Input: part model. Units: mm. Frame: model coordinates. A direction names the side the tool comes from. Give positions to 0.01 mm unless a question says otherwise; leave off trailing zeros. Write each loop counter-clockwise with the first axis right and the second up, starting at its lowest first coordinate (ties: lowest second). Pieces come first, ordered by that corner, then holes.
Autodesk Inventor part; units mm, degrees
ref_plane "YZ Plane" through (0, 0, 0) normal (1, 0, 0) x (0, 1, 0)
ref_plane "XZ Plane" through (0, 0, 0) normal (0, 1, 0) x (-1, 0, 0)
ref_plane "XY Plane" through (0, 0, 0) normal (0, 0, 1) x (1, 0, 0)
sketch "Sketch1" plane through (0, 0, 0) normal (0, 1, 0) x (-1, 0, 0)
  line L0 (25, 0) -> (-25, 0)
  line L1 (-25, 0) -> (-25, -3)
  line L2 (-25, -3) -> (25, -3)
  line L3 (25, -3) -> (25, 0)
  line L4 (0, 0) -> (0, -12.1399) construction
  line L5 (24.75, -3) -> (24.75, -17.6357)
  line L6 (18.75, -3) -> (18.75, -17.6357)
  arc A0 (18.75, -17.6357) -> (24.75, -17.6357) centre (21.75, -17.6357) ccw
  circle A1 centre (21.75, -17.6357) radius 1.85
  line L7 (-24.75, -3) -> (-24.75, -17.6357)
  line L8 (-18.75, -3) -> (-18.75, -17.6357)
  arc A2 (-24.75, -17.6357) -> (-18.75, -17.6357) centre (-21.75, -17.6357) ccw
  circle A3 centre (-21.75, -17.6357) radius 1.85
  line L9 (-24.75, -3) -> (-18.75, -3)
  dimension "d0" = 3
  dimension "d1" = 50
  dimension "d2" = 43.5
  dimension "d3" = 14.6357
  dimension "d4" = 3.7
  dimension "d5" = 3
extrude "Extrusion1" add sketch "Sketch1" along normal blind 15
sketch "Sketch2" plane through (-25, 0, 0) normal (0, 0, 1) x (1, 0, 0)
  line L0 (0, 0) -> (50, 0)
  line L1 (50, 0) -> (50, 15)
  line L2 (0, 15) -> (50, 15)
  line L3 (0, 0) -> (0, 15)
  circle A0 centre (15.5, 6.5) radius 3.25
  circle A1 centre (35.25, 7.4) radius 6
  line L4 (43.75, 0) -> (43.75, 15)
  point P0 (25, 0)
  point P1 (25, 0)
  point P2 (50, 7.5)
  point P3 (0, 7.5)
  dimension "d8" = 6.5
  dimension "d14" = 34.5
  dimension "d15" = 8.5
  dimension "d16" = 12
  dimension "d17" = 8.5
  dimension "d21" = 15
  dimension "d22" = 7.4
extrude "Extrusion2" cut sketch "Sketch2" against normal through all contours A0
sketch "Sketch3" plane through (0, 0, 0) normal (0, -1, 0) x (1, 0, 0)
  point P0 (0, 0)
extrude "Extrusion3" cut sketch "Sketch2" against normal through all contours A1
properties part number "portaswitch" material "Default New Material(1)"
Q1. Section B-B, the plane x = 10.25. Return the cut outline in (y, z), then the cut area to 3 significant figures.
Q2. Mould query, pull axis X, two halves, no side actions, for faces 3 (the cylindrical face through (-20.28, 7.4, -16.51)), 4 (the flat face through (24.75, 7, -10)), 5 (the flat face through (-24.75, 7, -10)), 6 (the flat face through (0, 7, 0)). Classes: +X half, -X half, draft (parallel to the pull), parting line (faces both ways), or undercut.
Q3. Material intervals for line 1 along Z through (x, y) = (21.75, 7.75); line 2 along X through (y, z) = (1.5, -4); line 3 along X through (y, z) = (5, -18.75), sorted ascending.
Q4. Section A-A, the plane z = -4. Return the cut outline in (x, y), then the cut area to 3 significant figures.
Q5. Section C-C, the plane y = 7.4. Return the cut outline in (x, z), then the cut area to 3 significant figures.
Q6. Section D-D, the plane y = 2. Return the cut outline in (x, z), then the cut area to 3 significant figures.
Q7. Pin query (flat end, axial travel): pin 1 (4 mm diameter, centred on y = 9, z = -16.5, fed in from +X); pin 2 (3 mm diameter, centred on y = 13, z = -7, fed in from -X); pin 3 (8 mm diameter, centred on x = 16, z = -10.5, fed in from +Y); pin 4 (12 mm diameter, centred on x = 6.5, z = -10.5, fed in from +Y). Return the tip coordinate at first contact, or that it passes through.
Q8. Access query for faces 1 (the flat face through (18.75, 7, -10)), 2 (the cylindrical face through (23.22, 7.4, -16.51)). Directions: +Z, -Z, +X, -X, +Y, -Y. A direction counts if a zero-diameter tool reaches every point of the face in a straight line with its end or side. Return the directions, or none.
Solutions:
1. outline: (0, -3) - (1.4, -3) - (1.4, 0) - (0, 0) - close; (13.4, -3) - (15, -3) - (15, 0) - (13.4, 0) - close
1. area: 9.00 mm2
2. face 3: undercut
2. face 4: +X half
2. face 5: -X half
2. face 6: draft
3. line 1: z = -20.64 to -19.49, -15.79 to 0
3. line 2: x = -24.75 to -18.75, 18.75 to 24.75
3. line 3: x = -24.54 to -23.23, -20.27 to -18.96, 18.96 to 20.27, 23.23 to 24.54
4. outline: (-24.75, 0) - (-18.75, 0) - (-18.75, 15) - (-24.75, 15) - close; (18.75, 0) - (24.75, 0) - (24.75, 15) - (18.75, 15) - close
4. area: 180 mm2
5. outline: (-25, -3) - (-24.75, -3) - (-24.75, -17.64) arc R3 ccw to (-18.75, -17.64) - (-18.75, -3) - (-12.62, -3) - (-12.62, 0) - (-25, 0) - close; (-6.38, -3) - (4.25, -3) - (4.25, 0) - (-6.38, 0) - close; (16.25, -3) - (18.75, -3) - (18.75, -17.64) arc R3 ccw to (24.75, -17.64) - (24.75, -3) - (25, -3) - (25, 0) - (16.25, 0) - close; hole circle Ø3.7 at (-21.75, -17.64); hole circle Ø3.7 at (21.75, -17.64)
5. area: 278 mm2
6. outline: (-25, -3) - (-24.75, -3) - (-24.75, -17.64) arc R3 ccw to (-18.75, -17.64) - (-18.75, -3) - (7.63, -3) - (7.63, 0) - (-25, 0) - close; (12.87, -3) - (18.75, -3) - (18.75, -17.64) arc R3 ccw to (24.75, -17.64) - (24.75, -3) - (25, -3) - (25, 0) - (12.87, 0) - close; hole circle Ø3.7 at (-21.75, -17.64); hole circle Ø3.7 at (21.75, -17.64)
6. area: 317 mm2
7. pin 1: stops at x = 24.75
7. pin 2: stops at x = -24.75
7. pin 3: stops at y = 15
7. pin 4: passes through
8. face 1: -Z, +Y, -Y
8. face 2: +Y, -Y
